```python
from build123d import *

# Parameters (mm, degrees)
F0_R     = 70.653692
F0_R_2   = 7.5
F1_DEPTH = 24.1


with BuildPart() as f1:
    # F0 (on Front) → F1 (new body)
    with BuildSketch(Plane.XZ):
        Circle(F0_R)
        with Locations((-27.966831, -45.815672)):
            Circle(F0_R_2, mode=Mode.SUBTRACT)
        with Locations((-49.555418, -20.627166)):
            Circle(F0_R_2, mode=Mode.SUBTRACT)
        with Locations((4.304135, -53.504148)):
            Circle(F0_R_2, mode=Mode.SUBTRACT)
        with Locations((34.931067, -40.755858)):
            Circle(F0_R_2, mode=Mode.SUBTRACT)
        with Locations((52.215519, -12.440216)):
            Circle(F0_R_2, mode=Mode.SUBTRACT)
        with Locations((-52.215519, 12.440216)):
            Circle(F0_R_2, mode=Mode.SUBTRACT)
        with Locations((-34.931067, 40.755858)):
            Circle(F0_R_2, mode=Mode.SUBTRACT)
        with Locations((-4.304135, 53.504148)):
            Circle(F0_R_2, mode=Mode.SUBTRACT)
        with Locations((49.555418, 20.627166)):
            Circle(F0_R_2, mode=Mode.SUBTRACT)
        with Locations((27.966831, 45.815672)):
            Circle(F0_R_2, mode=Mode.SUBTRACT)
    extrude(amount=F1_DEPTH)


solid = f1.part
```
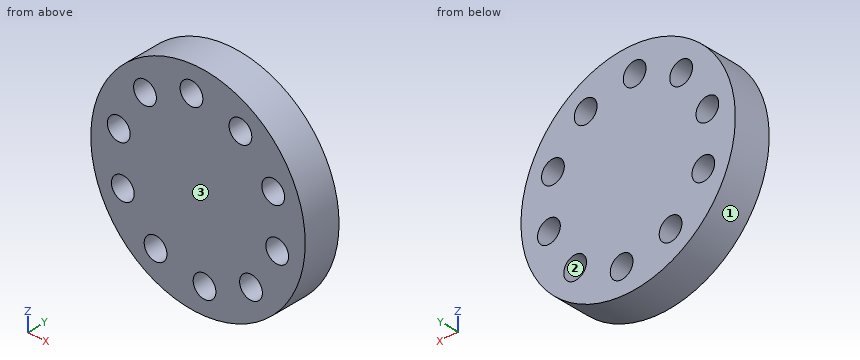
Input: part model. Units: mm. Frame: model coordinates. Face numbers are marked on the shaded views. Round coordinates to 2 decimals unless told otherwise and drop trailing zeros. Loops run counter-clockwise (first coordinate to the right, second up) from the corner with the lowest first, then second, coordinate; pieces in that order, holes last. Notation, with made-up numbers: (2.5, -39.75) - (27.5, -39.75) arc R11 ccw to (27.5, -28.75) - close; hole circle Ø3 at (45, 13). An arc over 180 degrees is marked (long way). One line per item, written item: value. Start each with the question number.
(1) Contact query for flat-ended pins moving along their axis: P1, Ø2, axis at x = 38, y = -3.5, coming from the +Z side; P2, Ø12, axis at y = -4.5, z = 35.5, coming from the +X side; P3, Ø10, axis at y = -18.5, z = -12, coming from the -X side. Output: stop coordinate, or through.
(2) Ray query, line 1 (X direction, y = -10.25, z = 49); line 2 (X direction, y = -20.75, z = -44.5); line 3 (Z direction, x = -28, y = -2.5). Return the intervals inside material, ascending. Write a range as [from, to].
(3) Section C-C, the plane x = 0. Return loops of the section in (y, z).
(4) Section D-D, the plane y = -7.5. Count the separate pieces of the cut face and the enclosed holes in it, plus the area to 3 significant figures.
(5) Draft query along Z for the marked faces 1, 2 and 3. Return one class per face: +Z half, -Z half, draft (parallel to the pull), parting line (faces both ways), or undercut.
(6) Section A-A, the plane z = 36. Return loops of the section in (x, y).
(7) Section B-B, the plane x = 38. Return loops of the section in (y, z).
Results below:
1. P1: z = 60.19
1. P2: x = 64.2
1. P3: x = -70.31
2. line 1: [-50.9, -10.3], [1.69, 21.18], [34.76, 50.9]
2. line 2: [-54.88, -35.35], [-20.58, 28.43], [41.43, 54.88]
2. line 3: [-64.87, -53.32], [-38.32, 37.89], [43.62, 64.87]
3. outline: (-24.1, -70.65) - (0, -70.65) - (0, -59.65) - (-24.1, -59.65) - close; (-24.1, -47.36) - (0, -47.36) - (0, 47.36) - (-24.1, 47.36) - close; (-24.1, 59.65) - (0, 59.65) - (0, 70.65) - (-24.1, 70.65) - close
4. separate pieces: 1
4. enclosed holes: 10
4. area: 13,900 mm^2
5. face 1: parting line
5. face 2: undercut
5. face 3: draft
6. outline: (-60.79, -24.1) - (-40.73, -24.1) - (-40.73, 0) - (-60.79, 0) - close; (-29.13, -24.1) - (60.79, -24.1) - (60.79, 0) - (-29.13, 0) - close
7. outline: (-24.1, -59.56) - (0, -59.56) - (0, -47.6) - (-24.1, -47.6) - close; (-24.1, -33.91) - (0, -33.91) - (0, 59.56) - (-24.1, 59.56) - close
